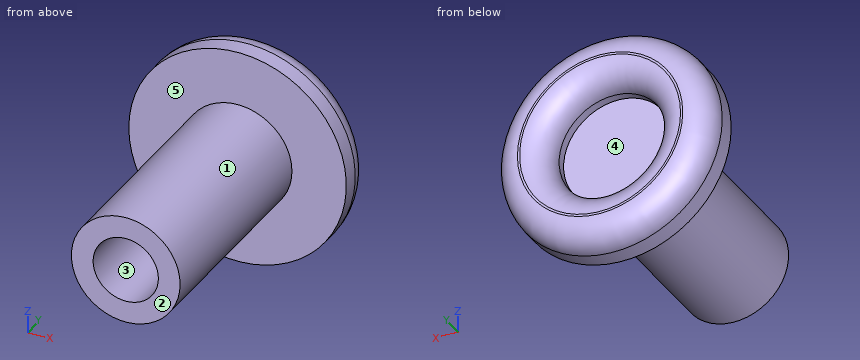
```python
from build123d import *

# Parameters (mm, degrees)
F0_R     = 1.5875
F1_DEPTH = 6.35
F2_R     = 0.9525
F3_DEPTH = 5.08
F4_R     = 3.175
F4_R_2   = 1.5875
F5_DEPTH = 1.27
F6_R     = 0.762
F7_DEPTH = 0.254


with BuildPart() as f1:
    # F0 (on Front) → F1 (new body)
    with BuildSketch(Plane.XZ):
        Circle(F0_R)
    extrude(amount=F1_DEPTH)

    # F2 (on face) → F3 (cut)
    with BuildSketch(Plane.XZ.offset(6.35)):
        Circle(F2_R)
    extrude(amount=-F3_DEPTH, mode=Mode.SUBTRACT)

    # F4 (on face) → F5 (join)
    with BuildSketch(Plane(origin=(0, 0, 0), x_dir=(-1, 0, 0), z_dir=(0, 1, 0))):
        Circle(F4_R)
        Circle(F4_R_2, mode=Mode.SUBTRACT)
    extrude(amount=F5_DEPTH)

    # F6
    f6_edges = [f1.edges().sort_by_distance(p)[0] for p in [
        (3.175, 1.27, 0),
        (1.5875, 1.27, 0),
    ]]
    fillet(f6_edges, radius=F6_R)

    # F7 (add): a face of the model
    f7_faces = [f1.faces().sort_by_distance(p)[0] for p in [
        (0, 0, 0),
    ]]
    extrude(f7_faces, amount=F7_DEPTH)


solid = f1.part
```
Check sheet for the modelled part. Datum: model origin and axes. Units: mm. Face numbers are marked on the shaded views. A direction names the side the tool comes from. Give positions to 0.01 mm unless a question says otherwise; leave off trailing zeros. Order: outer loops, then holes, each group sorted by start corner. A loop starts at its lowest first (then second) coordinate and runs counter-clockwise, first axis right, second up. Notation, with made-up numbers: (86.25, 75) -> (142.25, 75) arc R7 ccw to (142.25, 86) -> close; hole circle Ø7 at (-21, 68). An arc over 180 degrees is marked (long way). Return JSON: item names as keys, results as strings.
1. Material ranges on probe 1 along Z at (x, y) = (0, 0.45) (1 decimal); probe 2 along Y at (x, z) = (1.75, -1.5); probe 3 along Y at (x, z) = (0, -1), recorded low to high. Write a range as [from, to].
From the geometry:
{"probe 1": "[-3.2, -1.6], [1.6, 3.2]", "probe 2": "[0, 1.27]", "probe 3": "[-6.35, 0.25]"}
2. Cross-section at D-D, the plane y = -1. Record the cut outline in (x, z) (1 decimal), plus the area to 3 significant figures.
From the geometry:
{"outline": "circle Ø3.2 at (0, 0)", "area": "7.92 mm^2"}
3. Go/stop test with flat-tipped pins: P1, Ø3, axis at x = 2.5, z = 2.5, coming from the -Y side; P2, Ø1.6, axis at x = 0, z = 0, coming from the +Y side; P3, Ø1.5, axis at x = 0, z = 0, coming from the -Y side. Record where each tip stops, or that it passes through.
From the geometry:
{"P1": "y = 0", "P2": "y = 0.25", "P3": "y = -1.27"}
4. Mould release check, pull along Z, two halves, no side actions. Record for the marked faces 1, 2 and 3: +Z half, -Z half, draft (parallel to the pull), parting line (faces both ways), or undercut.
From the geometry:
{"face 1": "parting line", "face 2": "draft", "face 3": "undercut"}
5. Set-up check for the marked faces 4 and 5: record each of +Z, -Z, +X, -X, +Y, -Y from which the full face is reachable in a straight line by a thin tool's end or side.
From the geometry:
{"face 4": "+Y", "face 5": "-Y"}
6. Cross-section at C-C, the plane y = -4.5. Record the cut outline in (x, z) (1 decimal).
From the geometry:
{"outline": "circle Ø3.2 at (0, 0); hole circle Ø1.9 at (0, 0)"}
